```python
from build123d import *

# Parameters (mm, degrees)
EXTRUDE_1_DEPTH = 163
SKETCH_2_W      = 4.084844537
SKETCH_2_H      = 3.957854635
EXTRUDE_2_DEPTH = 2
SKETCH_3_W      = 4.4411109
SKETCH_3_H      = 4.15824399
EXTRUDE_3_DEPTH = 2
SKETCH_4_W      = 4.050772352
SKETCH_4_H      = 4.448077529
EXTRUDE_4_DEPTH = 2


with BuildPart() as part:
    # 草图1 → 凸台-拉伸1 (new body)
    with BuildSketch(Plane(origin=(0, 0, 0), x_dir=(1, 0, 0), z_dir=(0, 1, 0))):
        Polygon((0, -26.141443499), (-1.748690073, -26.141443499), (-1.748690073, -28.342387862), (0, -28.342387862), (0, -54), (-8, -54), (-8, 0), (0, 0), align=None)
    extrude(amount=-EXTRUDE_1_DEPTH)

    # 草图2 → 凸台-拉伸2 (add)
    with BuildSketch(Plane(origin=(0, 0, 0), x_dir=(-1, 0, 0), z_dir=(0, 0, -1))):
        with Locations((5.957577731, -20.96402105)):
            Rectangle(SKETCH_2_W, SKETCH_2_H)
    extrude(amount=EXTRUDE_2_DEPTH)

    # 草图3 → 凸台-拉伸3 (add)
    with BuildSketch(Plane(origin=(0, 0, 0), x_dir=(-1, 0, 0), z_dir=(0, 0, -1))):
        with Locations((5.77944455, -89.008990741)):
            Rectangle(SKETCH_3_W, SKETCH_3_H)
    extrude(amount=EXTRUDE_3_DEPTH)

    # 草图4 → 凸台-拉伸4 (add)
    with BuildSketch(Plane(origin=(0, 0, 0), x_dir=(-1, 0, 0), z_dir=(0, 0, -1))):
        with Locations((5.974613824, -143.08995755)):
            Rectangle(SKETCH_4_W, SKETCH_4_H)
    extrude(amount=EXTRUDE_4_DEPTH)


solid = part.part
```
Check sheet for the modelled part. Datum: model origin and axes. Units: mm. Round coordinates to 2 decimals unless told otherwise and drop trailing zeros. Loops run counter-clockwise (first coordinate to the right, second up) from the corner with the lowest first, then second, coordinate; pieces in that order, holes last. Notation, with made-up numbers: M 85,40 L 122,40 A24 cw 122,62 Z; hole C 38,89.5 d3. An arc over 180 degrees is marked long. Answer as a JSON object with one key per item and string values.
1. Section check C-C (y = -138.5). Record the boundary of the cut face in (x, z), plus the area to 3 significant figures.
Reply:
{"outline": "M -8,0 L 0,0 L 0,26.14 L -1.75,26.14 L -1.75,28.34 L 0,28.34 L 0,54 L -8,54 Z", "area": "428 mm²"}
2. Section check A-A (x = -5.25). Record the boundary of the cut face in (y, z).
Reply:
{"outline": "M -163,0 L -145.31,0 L -145.31,-2 L -140.87,-2 L -140.87,0 L -91.09,0 L -91.09,-2 L -86.93,-2 L -86.93,0 L -22.94,0 L -22.94,-2 L -18.99,-2 L -18.99,0 L 0,0 L 0,54 L -163,54 Z"}
3. Section check B-B (y = -89.5). Record the boundary of the cut face in (x, z).
Reply:
{"outline": "M -8,-2 L -3.56,-2 L -3.56,0 L 0,0 L 0,26.14 L -1.75,26.14 L -1.75,28.34 L 0,28.34 L 0,54 L -8,54 Z"}
4. Scan lines: line 1 (Z direction, x = -1.5, y = -96); line 2 (Z direction, x = -2.75, y = -128); line 3 (X direction, y = -20, z = 28). Record each from-to range of solid material in increasing order.
Reply:
{"line 1": "z = 0 to 26.14, 28.34 to 54", "line 2": "z = 0 to 54", "line 3": "x = -8 to -1.75"}
5. Gauge pin test, flat ends, axial feed: P1, Ø0.6, axis at x = -6.5, z = -1, coming from the +Y side; P2, Ø1, axis at x = -3, y = -118.5, coming from the -Z side; P3, Ø0.6, axis at x = -6, z = -0.5, coming from the -Y side. Record the tip position at first contact, or that the pin passes through.
Reply:
{"P1": "stops at y = -18.99", "P2": "stops at z = 0", "P3": "stops at y = -145.31"}
